Autodesk Inventor part; units mm, degrees
ref_plane "YZ Plane" through (0, 0, 0) normal (1, 0, 0) x (0, 1, 0)
ref_plane "XZ Plane" through (0, 0, 0) normal (0, 1, 0) x (-1, 0, 0)
ref_plane "XY Plane" through (0, 0, 0) normal (0, 0, 1) x (1, 0, 0)
sketch "Sketch1" plane through (0, 0, 0) normal (0, 0, 1) x (1, 0, 0)
  line L0 (0, 0) -> (25.4, 0)
  line L1 (25.4, 0) -> (25.4, 25.4)
  line L2 (25.4, 25.4) -> (0, 25.4)
  line L3 (0, 25.4) -> (0, 0)
  line L4 (1.5875, 23.8125) -> (23.8125, 23.8125)
  line L5 (23.8125, 23.8125) -> (23.8125, 1.5875)
  line L6 (23.8125, 1.5875) -> (1.5875, 1.5875)
  line L7 (1.5875, 1.5875) -> (1.5875, 23.8125)
  dimension "d0" = 25.4
  dimension "d1" = 25.4
  dimension "d2" = 1.5875
extrude "Extrusion1" add sketch "Sketch1" against normal blind 101.6
sketch "Sketch3" plane through (0, 0, 0) normal (0, -1, 0) x (1, 0, 0)
  line L0 (0, -101.6) -> (25.4, -101.6)
  line L1 (0, 0) -> (25.4, 0)
  point P0 (12.7, -12.7)
  point P1 (12.7, -88.9)
  dimension "d7" = 12.7
  dimension "d8" = 12.7
hole "Hole2" at (12.7, 0, -12.7) at (12.7, 0, -88.9) direction (0, 1, 0) diameter 6.35 depth 25.4 tip angle 118
properties part number "tube_r_f_in"
The listing builds one solid part. Answer for the finished solid, in the listing's coordinates (mm). A direction names the side the tool comes from. Coordinates: 2 decimals unless noted, no trailing zeros. Loops run counter-clockwise (first coordinate to the right, second up) from the corner with the lowest first, then second, coordinate; pieces in that order, holes last. Notation, with made-up numbers: M 64,78 L 115,78 A21 ccw 115,93 Z; hole C -6.75,37.5 d3. An arc over 180 degrees is marked long. Answer in a Markdown table with one row per item.
1) Find section B-B (z = -12.7). Determine the outline of the cut face in (x, y) (1 decimal).
Answers below:
| item | result |
|---|---|
| outline | M 0,0 L 9.5,0 L 9.5,1.6 L 1.6,1.6 L 1.6,23.8 L 9.5,23.8 L 9.5,25.4 L 0,25.4 Z; M 15.9,0 L 25.4,0 L 25.4,25.4 L 15.9,25.4 L 15.9,23.8 L 23.8,23.8 L 23.8,1.6 L 15.9,1.6 Z |
2) Find section C-C (x = 20.25). Determine the outline of the cut face in (y, z), then the cut area to 3 significant figures.
Answers below:
| item | result |
|---|---|
| outline | M 0,-101.6 L 1.59,-101.6 L 1.59,0 L 0,0 Z; M 23.81,-101.6 L 25.4,-101.6 L 25.4,0 L 23.81,0 Z |
| area | 323 mm^2 |
3) Determine the mould class of faces 1 (the flat face through (1, 13, -101.6)), 2 (the cylindrical face through (14.63, 24.62, -86.38)), 3 (the flat face through (13, 0, -50)), 4 (the cylindrical face through (14.63, 0.8, -10.18)) for opening direction Z: released by +Z, released by -Z, zero draft, split by the parting line, or undercut.
Answers below:
| item | result |
|---|---|
| face 1 | released by -Z |
| face 2 | undercut |
| face 3 | zero draft |
| face 4 | undercut |
4) Find the intervals of material crossed by probe 1 along Z at (x, y) = (12.7, 1.2) (3 decimals); probe 2 along Y at (x, z) = (14.5, -42); probe 3 along X at (y, z) = (24.6, -12.7) (3 decimals), in increasing order.
Answers below:
| item | result |
|---|---|
| probe 1 | -101.6 to -92.075, -85.725 to -15.875, -9.525 to 0 |
| probe 2 | 0 to 1.59, 23.81 to 25.4 |
| probe 3 | 0 to 9.525, 15.875 to 25.4 |
5) Given pin 1 (6.5 mm diameter, centred on x = 8.5, z = -63, fed in from -Y), flat-ended and moving along its own axis, determine where the tip first touches the part or whether it passes through.
Answers below:
| item | result |
|---|---|
| pin 1 | y = 0 |
6) Find section A-A (x = 12.7). Determine the outline of the cut face in (y, z) (1 decimal), then the cut area to 3 significant figures.
Answers below:
| item | result |
|---|---|
| outline | M 0,-101.6 L 1.6,-101.6 L 1.6,-92.1 L 0,-92.1 Z; M 0,-85.7 L 1.6,-85.7 L 1.6,-15.9 L 0,-15.9 Z; M 0,-9.5 L 1.6,-9.5 L 1.6,0 L 0,0 Z; M 23.8,-101.6 L 25.4,-101.6 L 25.4,-92.1 L 23.8,-92.1 Z; M 23.8,-85.7 L 25.4,-85.7 L 25.4,-15.9 L 23.8,-15.9 Z; M 23.8,-9.5 L 25.4,-9.5 L 25.4,0 L 23.8,0 Z |
| area | 282 mm^2 |
7) Which of the six approach directions +Z, -Z, +X, -X, +Y, -Y give full straight-line access (tool end or side, diameter ignored) to faces 5 (the flat face through (13, 25.4, -50)), 6 (the flat face through (23.812, 13, -50))?
Answers below:
| item | result |
|---|---|
| face 5 | +Z, -Z, +X, -X, +Y |
| face 6 | +Z, -Z |
8) Find section D-D (z = -71). Determine the outline of the cut face in (x, y).
Answers below:
| item | result |
|---|---|
| outline | M 0,0 L 25.4,0 L 25.4,25.4 L 0,25.4 Z; hole M 1.59,1.59 L 23.81,1.59 L 23.81,23.81 L 1.59,23.81 Z |
